Design review of the part built by this model. Coordinates are the model's own, in mm. Face numbers are marked on the shaded views. A direction names the side the tool comes from. Coordinates: 2 decimals unless noted, no trailing zeros. Write each loop counter-clockwise with the first axis right and the second up, starting at its lowest first coordinate (ties: lowest second). Pieces come first, ordered by that corner, then holes. Notation, with made-up numbers: (41, 35) - (82, 35) arc R15 ccw to (82, 52) - close; hole circle Ø6 at (69, 84). An arc over 180 degrees is marked (long way). Answer as CSV lines item,"result". Start each with the question number.
Q1. We need section C-C (x = 78). Write out the cut boundary in (y, z).
Q2. Machinability: for the marked faces 1, 2 and 3, which of the approach directions +Z, -Z, +X, -X, +Y, -Y give a long, thin tool a straight path to every point of the face, cutting with its end or side? Answer none if there is none.
Q3. Clearance check with flat-ended pins moving along their axes: pin 1 (2 mm diameter, centred on x = 66, z = 1.5, fed in from +Y); pin 2 (3 mm diameter, centred on x = 38, z = 5, fed in from +Y); pin 3 (3 mm diameter, centred on x = 60, z = 5, fed in from +Y); pin 4 (3 mm diameter, centred on x = 77, y = 82, fed in from +Z). State where each tip first meets the part, or that it passes through.
Q4. Mouldability with a two-part tool opening along Y and no side actions: class the marked faces 4, 5, 6 and 7 as pulls with the +Y half, pulls with the -Y half, needs draft (parallel to the pull), parting line crosses it, or undercut.
Q5. For line 1 along X through (y, z) = (36.5, 4); line 2 along X through (y, z) = (39.5, 2.5); line 3 along Y through (x, z) = (45, 4.5), list the stretches that pass through material, from the lowest coordinate up. Write a range as [from, to].
Q6. We need section D-D (y = 36.5). Write out the cut boundary in (x, z), plus the area to 3 significant figures.
Q7. We need section A-A (z = 4). State how many separate pieces and enclosed holes the cut face has, plus the area to 3 significant figures.
Q8. We need section B-B (y = 59). Write out the cut boundary in (x, z).
from build123d import *

# Parameters (mm, degrees)
F0_R     = 4.7625
F1_DEPTH = 9.7028


with BuildPart() as f1:
    # F0 (on Top) → F1 (new body)
    with BuildSketch(Plane.XY):
        with BuildLine():
            ThreePointArc((25.317648, 48.26209), (12.617648, 35.56209), (25.317648, 22.86209))
            Line((25.317648, 22.86209), (76.117648, 22.86209))
            ThreePointArc((76.117648, 22.86209), (85.097904, 26.581834), (88.817648, 35.56209))
            Line((88.817648, 35.56209), (88.817648, 86.36209))
            ThreePointArc((88.817648, 86.36209), (85.097904, 95.342346), (76.117648, 99.06209))
            ThreePointArc((76.117648, 99.06209), (67.137391, 95.342346), (63.417648, 86.36209))
            Line((63.417648, 86.36209), (63.417648, 60.96209))
            ThreePointArc((63.417648, 60.96209), (59.697904, 51.981834), (50.717648, 48.26209))
            Line((50.717648, 48.26209), (25.317648, 48.26209))
        make_face()
        with Locations((25.317648, 35.56209)):
            Circle(F0_R, mode=Mode.SUBTRACT)
        with BuildLine():
            Line((79.292648, 60.96209), (79.292648, 38.73709))
            ThreePointArc((79.292648, 38.73709), (77.432776, 34.246962), (72.942648, 32.38709))
            Line((72.942648, 32.38709), (50.717648, 32.38709))
            ThreePointArc((50.717648, 32.38709), (47.542648, 35.56209), (50.717648, 38.73709))
            Line((50.717648, 38.73709), (66.592648, 38.73709))
            ThreePointArc((66.592648, 38.73709), (71.082776, 40.596962), (72.942648, 45.08709))
            Line((72.942648, 45.08709), (72.942648, 60.96209))
            ThreePointArc((72.942648, 60.96209), (76.117648, 64.13709), (79.292648, 60.96209))
        make_face(mode=Mode.SUBTRACT)
        with BuildLine():
            ThreePointArc((72.942648, 82.812332), (74.173365, 90.709638), (80.880148, 86.36209))
            ThreePointArc((80.880148, 86.36209), (80.465195, 84.417808), (79.292648, 82.812332))
            ThreePointArc((79.292648, 82.812332), (76.117648, 81.59959), (72.942648, 82.812332))
        make_face(mode=Mode.SUBTRACT)
    extrude(amount=F1_DEPTH)


solid = f1.part
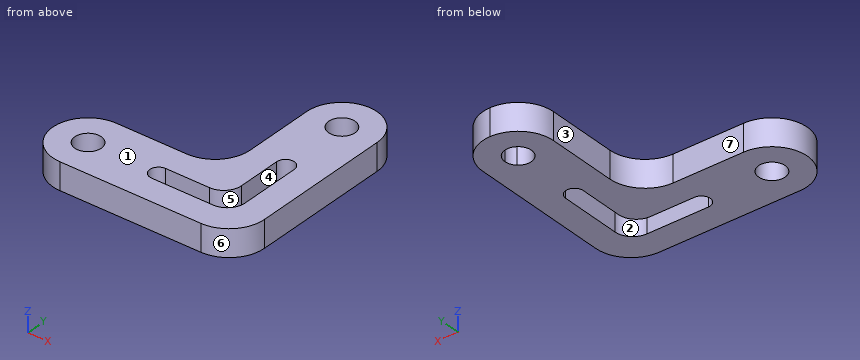
Results list:
1,outline,"(23, 0) - (34.9, 0) - (34.9, 9.7) - (23, 9.7) - close; (63.52, 0) - (81.99, 0) - (81.99, 9.7) - (63.52, 9.7) - close; (90.74, 0) - (98.92, 0) - (98.92, 9.7) - (90.74, 9.7) - close"
2,face 1,"+Z, +X, -X, +Y, -Y"
2,face 2,"+Z, -Z"
2,face 3,"+Z, -Z, -X, +Y"
3,pin 1,"stops at y = 95.2"
3,pin 2,"stops at y = 48.26"
3,pin 3,"stops at y = 54.25"
3,pin 4,"stops at z = 9.7"
4,face 4,"undercut"
4,face 5,"undercut"
4,face 6,"pulls with the -Y half"
4,face 7,"pulls with the +Y half"
5,line 1,"x = [12.65, 20.65], [29.99, 47.68], [78.89, 88.82]"
5,line 2,"x = [13.24, 22.64], [28, 69.61], [79.29, 88.82]"
5,line 3,"y = [22.86, 48.26]"
6,outline,"(12.65, 0) - (20.65, 0) - (20.65, 9.7) - (12.65, 9.7) - close; (29.99, 0) - (47.68, 0) - (47.68, 9.7) - (29.99, 9.7) - close; (78.89, 0) - (88.82, 0) - (88.82, 9.7) - (78.89, 9.7) - close"
6,area,"346 mm2"
7,separate pieces,"1"
7,enclosed holes,"3"
7,area,"2,590 mm2"
8,outline,"(63.27, 0) - (72.94, 0) - (72.94, 9.7) - (63.27, 9.7) - close; (79.29, 0) - (88.82, 0) - (88.82, 9.7) - (79.29, 9.7) - close"
